Part model, mm, in its own coordinate system. A direction names the side the tool comes from. Give positions to 0.01 mm unless a question says otherwise; leave off trailing zeros. Order: outer loops, then holes, each group sorted by start corner. A loop starts at its lowest first (then second) coordinate and runs counter-clockwise, first axis right, second up. Notation, with made-up numbers: (39.25, 1) - (65.25, 1) arc R9 cw to (65.25, 9) - close; hole circle Ø1 at (-27.5, 56). An arc over 180 degrees is marked (long way). Use a Markdown table: item, result. Add a question column.
Autodesk Fusion 360 part; units mm, degrees
sketch "Sketch1" plane through (0, 0, 0) normal (0, 0, 1) x (1, 0, 0)
  line L0 (0, 0) -> (6.35, 0)
  line L1 (6.35, 0) -> (6.35, 1.95)
  line L2 (6.35, 1.95) -> (1.95, 1.95)
  line L3 (0, 4.3112) -> (0, 0)
  line L4 (0, 0) -> (5, 0)
  line L5 (1.95, 1.95) -> (1.95, 5)
  line L6 (1.95, 5) -> (0, 5)
  line L7 (0, 5) -> (0, 0)
  dimension "d1" = 1.95
  dimension "d2" = 1.95
  dimension "d5" = 4.4
  dimension "d6" = 3.05
extrude "Extrude1" add sketch "Sketch1" along normal blind 7
sketch "Sketch2" plane through (0, 0, 0) normal (0, -1, 0) x (1, 0, 0)
  line L0 (0, 0) -> (6.35, 0)
  line L1 (6.35, 0) -> (6.35, 7)
  line L2 (6.35, 7) -> (0, 7)
  line L3 (0, 7) -> (0, 0)
  line L4 (6.35, 7) -> (-1.55, 7)
  line L5 (-1.55, 7) -> (-1.55, 5)
  line L6 (-1.55, 5) -> (6.35, 5)
  line L7 (6.35, 5) -> (6.35, 7)
  dimension "d9" = 2
  dimension "d10" = 7.9
extrude "Extrude2" add sketch "Sketch2" along normal blind 8 contours L3 L4 L5 L6 | L1 L2 L3 L4 L6 L7
sketch "Sketch3" plane through (0, 0, 7) normal (0, 0, 1) x (-1, 0, 0)
  line L0 (0, -5) -> (0, 0)
  line L1 (0, 0) -> (1.55, 0)
  line L2 (1.55, 0) -> (1.55, 8)
  line L3 (1.55, 8) -> (-6.35, 8)
  line L4 (-6.35, 8) -> (-6.35, -1.95)
  line L5 (-6.35, -1.95) -> (-1.95, -1.95)
  line L6 (-1.95, -1.95) -> (-1.95, -5)
  line L7 (-1.95, -5) -> (0, -5)
  circle A0 centre (-2.45, 4) radius 1.5
  dimension "d14" = 4
  dimension "d15" = 4
  dimension "d16" = 3
extrude "Extrude3" cut sketch "Sketch3" against normal blind 4 contours A0
1. Cut at D-D (z = 4.5). Write the cut outline in (x, y), plus the area to 3 significant figures.
2. Tool access for faces 1 (the face through (-1.55, -4, 6)), 2 (the face through (4, 1.95, 3)), 3 (the face through (2, 1, 0)), 4 (the face through (0, 3, 3)), 5 (the face through (3, 0, 2)): list every direction of +Z, -Z, +X, -X, +Y, -Y with a clear straight run to the whole face (end or side of a thin tool).
3. Cut at B-B (x = 2.45). Write the cut outline in (y, z).
4. Mould opens along Y. For faces 6 (the face through (0.6, -3.9, 5)), 7 (the face through (3.56, -5.01, 6.01)), 8 (the face through (-1, 0, 6)), 9 (the face through (2, -8, 6)) say: released by +Y, released by -Y, zero draft, split by the parting line, or undercut.
5. Cut at C-C (y = -4). Write the cut outline in (x, z).
6. Cut at A-A (z = 6). Write the cut outline in (x, y).
7. Pin check, flat tips, straight feed: P1, Ø3.5, axis at x = 2.45, y = -4, coming from the -Z side; P2, Ø4, axis at y = 3, z = 5, coming from the -X side; P3, Ø2, axis at x = 3.5, z = 2.5, coming from the +Y side. Stop position of each tip, or through.
8. Drill centre lines: probe 1 along X at (y, z) = (-4, 6.25); probe 2 along Y at (x, z) = (2.45, 6); probe 3 along Z at (x, y) = (5, -1.5). Where is each one in solid material? Low to high. Write a range as [from, to].
Responses:
| question | item | result |
|---|---|---|
| 1 | outline | (0, 0) - (6.35, 0) - (6.35, 1.95) - (1.95, 1.95) - (1.95, 5) - (0, 5) - close |
| 1 | area | 18.3 mm² |
| 2 | face 1 | +Z, -Z, -X, +Y, -Y |
| 2 | face 2 | +Z, -Z, +X, +Y |
| 2 | face 3 | -Z, +X, -X, +Y, -Y |
| 2 | face 4 | +Z, -Z, -X, +Y |
| 2 | face 5 | -Z, +X, -X, -Y |
| 3 | outline | (-8, 5) - (-5.5, 5) - (-5.5, 7) - (-8, 7) - close; (-2.5, 5) - (0, 5) - (0, 0) - (1.95, 0) - (1.95, 7) - (-2.5, 7) - close |
| 4 | face 6 | zero draft |
| 4 | face 7 | undercut |
| 4 | face 8 | released by +Y |
| 4 | face 9 | released by -Y |
| 5 | outline | (-1.55, 5) - (0.95, 5) - (0.95, 7) - (-1.55, 7) - close; (3.95, 5) - (6.35, 5) - (6.35, 7) - (3.95, 7) - close |
| 6 | outline | (-1.55, -8) - (6.35, -8) - (6.35, 1.95) - (1.95, 1.95) - (1.95, 5) - (0, 5) - (0, 0) - (-1.55, 0) - close; hole circle Ø3 at (2.45, -4) |
| 7 | P1 | stops at z = 5 |
| 7 | P2 | stops at x = 0 |
| 7 | P3 | stops at y = 1.95 |
| 8 | probe 1 | x = [-1.55, 0.95], [3.95, 6.35] |
| 8 | probe 2 | y = [-8, -5.5], [-2.5, 1.95] |
| 8 | probe 3 | z = [5, 7] |
